Geometry: final body of the model. Coordinates: model frame, mm. Coordinates: 2 decimals unless noted, no trailing zeros. Order: outer loops, then holes, each group sorted by start corner. A loop starts at its lowest first (then second) coordinate and runs counter-clockwise, first axis right, second up. Notation, with made-up numbers: (-37, 78) -> (-18, 78) arc R34 ccw to (-18, 110) -> close; hole circle Ø1 at (-26, -19). An arc over 180 degrees is marked (long way). Use one line per item in the form item = value.
```python
from build123d import *

# Parameters (mm, degrees)
SKETCH1_R           = 8.25
BOSS_EXTRUDE1_DEPTH = 15
FILLET1_R           = 10
BOSS_EXTRUDE2_DEPTH = 15
SKETCH3_W           = 20
SKETCH3_H           = 25
CUT_EXTRUDE1_DEPTH  = 262.971372482
FILLET2_R           = 10
SKETCH4_R           = 2
CUT_EXTRUDE2_DEPTH  = 262.971372482


with BuildPart() as part:
    # Sketch1 → Boss-Extrude1 (new body)
    with BuildSketch(Plane(origin=(0, 0, 0), x_dir=(1, 0, 0), z_dir=(0, 1, 0))):
        Polygon((-105, 0), (105, 0), (105, 70), (95, 70), (60, 30), (-60, 30), (-95, 70), (-105, 70), align=None)
        with Locations(Location((0, 17.15, 0), (0, 0, 270))):
            Circle(SKETCH1_R, mode=Mode.SUBTRACT)
    extrude(amount=BOSS_EXTRUDE1_DEPTH)

    # Fillet1
    fillet1_edges = [part.edges().sort_by_distance(p)[0] for p in [
        (-95, 7.5, -70),
        (-60, 7.5, -30),
        (60, 7.5, -30),
        (95, 7.5, -70),
    ]]
    fillet(fillet1_edges, radius=FILLET1_R)

    # Sketch2 → Boss-Extrude2 (add)
    with BuildSketch(Plane(origin=(0, 15, 0), x_dir=(1, 0, 0), z_dir=(0, 1, 0))):
        Polygon((105, 0), (252, 0), (252, 45), (120.5, 45), (120.5, 30), (105, 30), align=None)
    boss_extrude2 = extrude(amount=-BOSS_EXTRUDE2_DEPTH)

    # Mirror1: Boss-Extrude2 across plane
    add(boss_extrude2.mirror(Plane(origin=(0, 0, 0), x_dir=(0, 0, 1), z_dir=(1, 0, 0))))

    # Sketch3 → Cut-Extrude1 (cut, through all)
    with BuildSketch(Plane(origin=(0, 15, 0), x_dir=(1, 0, 0), z_dir=(0, 1, 0))):
        with Locations((83, 12.5)):
            Rectangle(SKETCH3_W, SKETCH3_H)
    extrude(amount=-CUT_EXTRUDE1_DEPTH, mode=Mode.SUBTRACT)

    # Fillet2
    fillet2_edges = [part.edges().sort_by_distance(p)[0] for p in [
        (73, 7.5, -25),
        (93, 7.5, -25),
    ]]
    fillet(fillet2_edges, radius=FILLET2_R - 0.0001)  # a hair under: the kernel refuses the full size

    # Sketch4 → Cut-Extrude2 (cut, through all)
    with BuildSketch(Plane(origin=(0, 15, 0), x_dir=(1, 0, 0), z_dir=(0, 1, 0))):
        with Locations((-119.792893219, 30.707106781)):
            Circle(SKETCH4_R)
        with Locations((-105.707106781, 30.707106781)):
            Circle(SKETCH4_R)
        with Locations((105.707106781, 30.707106781)):
            Circle(SKETCH4_R)
        with Locations((119.792893219, 30.707106781)):
            Circle(SKETCH4_R)
    extrude(amount=-CUT_EXTRUDE2_DEPTH, mode=Mode.SUBTRACT)


solid = part.part
```
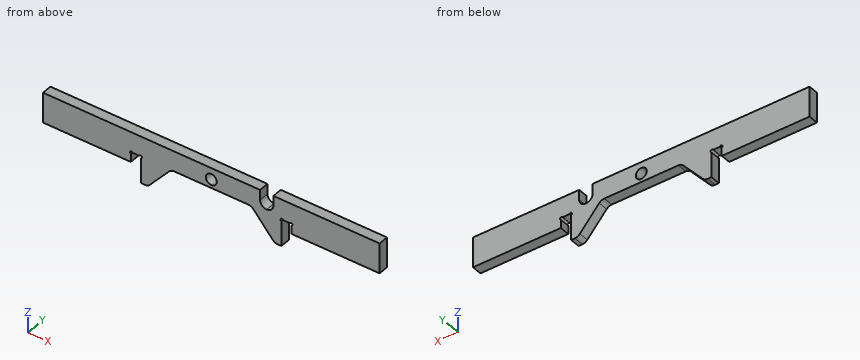
1) Material intervals for probe 1 along X at (y, z) = (8.5, -17.15); probe 2 along X at (y, z) = (1, -43.5); probe 3 along X at (y, z) = (6, -13), sorted ascending. Write a range as from..to.
Results found:
probe_1 = -252..-8.25, 8.25..73.23, 92.77..252
probe_2 = -252..-120.5, -105..-71.81, 71.81..105, 120.5..252
probe_3 = -252..-7.13, 7.13..73, 93..252
2) Contact query for flat-ended pins moving along their axis: P1, Ø1.5, axis at y = 3, z = -49.5, coming from the -X side; P2, Ø3, axis at y = 2, z = -57, coming from the +X side; P3, Ø4.5, axis at x = 197, y = 9, coming from the -Z side. Output: stop coordinate, or through.
Results found:
P1 = -105
P2 = 105
P3 = -45
3) Section C-C, the plane z = -59.5. Output: boundary loops of the cut face in (x, y).
Results found:
outline = (-105, 0) -> (-85.81, 0) -> (-85.81, 15) -> (-105, 15) -> close; (85.81, 0) -> (105, 0) -> (105, 15) -> (85.81, 15) -> close
4) Section D-D, the plane x = 181. Output: boundary loops of the cut face in (y, z), and give its area (3 significant figures).
Results found:
outline = (0, -45) -> (15, -45) -> (15, 0) -> (0, 0) -> close
area = 675 mm2
5) Section A-A, the plane x = 0. Output: boundary loops of the cut face in (y, z), and give its area (4 significant figures).
Results found:
outline = (0, -30) -> (15, -30) -> (15, -25.4) -> (0, -25.4) -> close; (0, -8.9) -> (15, -8.9) -> (15, 0) -> (0, 0) -> close
area = 202.5 mm2
